Build history of the part. All positions in model axes, mm. A direction names the side the tool comes from. Round coordinates to 2 decimals unless told otherwise and drop trailing zeros. Order: outer loops, then holes, each group sorted by start corner. A loop starts at its lowest first (then second) coordinate and runs counter-clockwise, first axis right, second up. Notation, with made-up numbers: (55, 89) -> (90, 89) arc R23 ccw to (90, 116) -> close; hole circle Ø3 at (29.25, 59.25). An arc over 180 degrees is marked (long way). Use a Markdown table: item, result. Add a question column.
Item 1: Pin check, flat tips, straight feed: pin 1 (3 mm diameter, centred on y = -1.5, z = 4.5, fed in from -X); pin 2 (2 mm diameter, centred on x = 5, z = 4.5, fed in from -Y). Stop position of each tip, or through.
Item 2: Probe L1, parallel to X at y = -1.25, z = 0.75; L2, parallel to X at y = -2.25, z = -1.75; L3, parallel to Z at x = 1, y = -3.5. List the from-to ranges inside material, lowest first.
Item 3: Slice it at A-A, the plane x = -7. Give the cut face in (y, z) (3 decimals).
Item 4: Slice it at C-C, the plane y = -1. State how many separate pieces and enclosed holes the cut face has, plus the area to 3 significant figures.
Item 5: Slice it at B-B, the plane z = 3.75. Give the cut face in (x, y), plus the area to 3 significant figures.
Item 6: 3-axis set-ups, long thin cutter, end or side, ignore diameter. For faces 4 (the face through (-8.24, -1.97, 6.1)), 5 (the face through (-1.35, -3.289, 1.375)), 6 (the face through (-8.223, -1.972, -6.114)): which of +Z, -Z, +X, -X, +Y, -Y reach the whole face in a straight line?
Item 7: Two-plate mould, pull along Z, no slides. Class faces 1 (the face through (-2, -0.5, 1)), 2 (the face through (8.223, -1.972, 6.114)), 3 (the face through (2, -6, 0)): released by +Z, released by -Z, zero draft, split by the parting line, or undercut.
from build123d import *

# Parameters (mm, degrees)
BOSS_EXTRUDE1_DEPTH = 4
BOSS_EXTRUDE1_DRAFT = 1
SHELL1_T            = -0.5
SKETCH2_R           = 2
BOSS_EXTRUDE2_DEPTH = 5.5
BOSS_EXTRUDE2_TAPER = 1.5
CIRPATTERN1_COUNT   = 4
SKETCH4_R           = 1.605977431
CUT_EXTRUDE1_DEPTH  = 5.5
CUT_EXTRUDE1_DRAFT  = 1.5
BOSS_EXTRUDE3_DEPTH = 2.5
BOSS_EXTRUDE4_DEPTH = 2.5


with BuildPart() as part:
    # Sketch1 → Boss-Extrude1 (with draft: the straight prism first)
    with BuildSketch(Plane(origin=(0, 0, 0), x_dir=(1, 0, 0), z_dir=(0, 1, 0))):
        with BuildLine():
            Line((-7.5, -6.375), (7.5, -6.375))
            ThreePointArc((7.5, -6.375), (8.207106781, -6.082106781), (8.5, -5.375))
            Line((8.5, -5.375), (8.5, 5.375))
            ThreePointArc((8.5, 5.375), (8.207106781, 6.082106781), (7.5, 6.375))
            Line((7.5, 6.375), (-7.5, 6.375))
            ThreePointArc((-7.5, 6.375), (-8.207106781, 6.082106781), (-8.5, 5.375))
            Line((-8.5, 5.375), (-8.5, -5.375))
            ThreePointArc((-8.5, -5.375), (-8.207106781, -6.082106781), (-7.5, -6.375))
        make_face()
    extrude(amount=-BOSS_EXTRUDE1_DEPTH)
    # Boss-Extrude1: the draft: its side faces are tilted about the plane it starts from
    boss_extrude1_sides = [part.faces().sort_by_distance(p)[0] for p in [
        (0, -2, 6.375),
        (8.207106781, -2, 6.082106781),
        (8.5, -2, 0),
        (8.207106781, -2, -6.082106781),
        (0, -2, -6.375),
        (-8.207106781, -2, -6.082106781),
        (-8.5, -2, 0),
        (-8.207106781, -2, 6.082106781),
    ]]
    draft(boss_extrude1_sides, Plane(origin=(0, 0, 0), x_dir=(1, 0, 0), z_dir=(0, 1, 0)), BOSS_EXTRUDE1_DRAFT)

    # Shell1
    shell1_openings = [part.faces().sort_by_distance(p)[0] for p in [
        (0, -4, 0),
    ]]
    offset(amount=SHELL1_T, openings=shell1_openings, kind=Kind.INTERSECTION)

    # Sketch2 → Boss-Extrude2 (add)
    with BuildSketch(Plane.XZ.offset(0.5)):
        Circle(SKETCH2_R)
    extrude(amount=BOSS_EXTRUDE2_DEPTH, taper=BOSS_EXTRUDE2_TAPER)

    # Rib1: read off the stored shape, not the designer's step
    # Rib1: loft between two sections, ruled curve by curve
    rib1_from = [
        Edge.make_line((1.982008415, -0.5, 0.267661433), (3, -0.5, 0.25)),
        Edge.make_line((1.982008415, -0.5, -0.267661433), (3, -0.5, -0.25)),
        Edge.make_line((3, -0.5, -0.25), (3, -0.5, 0.25)),
        Edge.make_line((1.982008415, -0.5, -0.267661433), (1.982008415, -0.5, 0.267661433)),
    ]
    rib1_to = [
        Edge.make_line((1.837730654, -6, 0.259611763), (2.391745366, -6, 0.25)),
        Edge.make_line((1.837730654, -6, -0.259611763), (2.391745366, -6, -0.25)),
        Edge.make_line((2.391745366, -6, -0.25), (2.391745366, -6, 0.25)),
        Edge.make_line((1.837730654, -6, -0.259611763), (1.837730654, -6, 0.259611763)),
    ]
    rib1 = Solid(Shell([*[Face.make_surface_from_curves(rib1_from[k], rib1_to[k]) for k in range(4)], Face(Wire(rib1_from)), Face(Wire(rib1_to))]))
    add(rib1)

    # CirPattern1: Rib1 ×4 about axis
    cirpattern1_axis = Axis((0, 0, 0), (0, 1, 0))
    for i in range(1, CIRPATTERN1_COUNT):
        add(rib1.rotate(cirpattern1_axis, i * 360 / CIRPATTERN1_COUNT))


with BuildPart() as cut_extrude1_tool:
    # Sketch4 → Cut-Extrude1 (with draft: the straight prism first)
    with BuildSketch(Plane.XZ.offset(6)):
        Circle(SKETCH4_R)
    extrude(amount=-CUT_EXTRUDE1_DEPTH)
    # Cut-Extrude1: the draft: its side faces are tilted about the plane it starts from
    cut_extrude1_sides = [cut_extrude1_tool.faces().sort_by_distance(p)[0] for p in [
        (-1.605977431, -3.25, 0),
    ]]
    draft(cut_extrude1_sides, Plane.XZ.offset(6), CUT_EXTRUDE1_DRAFT)


with BuildPart() as part_1:
    add(part.part)

    # Cut-Extrude1: cut by cut_extrude1_tool
    add(cut_extrude1_tool.part, mode=Mode.SUBTRACT)

    # Sketch5 → Boss-Extrude3 (add, symmetric)
    with BuildSketch(Plane(origin=(0, 0, 0), x_dir=(0, 0, -1), z_dir=(1, 0, 0))):
        Polygon((6.44482026, -4), (6.40991013, -2), (6.70991013, -2), align=None)
        Polygon((-6.70991013, -2), (-6.44482026, -4), (-6.40991013, -2), align=None)
    extrude(amount=BOSS_EXTRUDE3_DEPTH, both=True)

    # Sketch6 → Boss-Extrude4 (add, symmetric)
    with BuildSketch(Plane.XY):
        Polygon((8.56982026, -4), (8.53491013, -2), (8.83491013, -2), align=None)
        Polygon((-8.83491013, -2), (-8.56982026, -4), (-8.53491013, -2), align=None)
    extrude(amount=BOSS_EXTRUDE4_DEPTH, both=True)


solid = part_1.part
Check sheet entries:
| question | item | result |
|---|---|---|
| 1 | pin 1 | x = -8.55 |
| 1 | pin 2 | y = -0.5 |
| 2 | L1 | -8.52 to -8.02, -1.83 to -1.56, 1.56 to 1.83, 8.02 to 8.52 |
| 2 | L2 | -8.8 to -8.04, -0.87 to 0.87, 8.04 to 8.8 |
| 2 | L3 | -6.51 to -5.94, -1.64 to -1.34, 1.34 to 1.64, 5.94 to 6.51 |
| 3 | outline | (-4, -6.445) -> (0, -6.375) -> (0, 6.375) -> (-4, 6.445) -> (-4, 5.945) -> (-0.5, 5.884) -> (-0.5, -5.884) -> (-4, -5.945) -> close |
| 4 | separate pieces | 2 |
| 4 | enclosed holes | 2 |
| 4 | area | 33.1 mm2 |
| 5 | outline | (-8.57, -4) -> (-8.07, -4) -> (-8.01, -0.5) -> (8.01, -0.5) -> (8.07, -4) -> (8.57, -4) -> (8.5, 0) -> (-8.5, 0) -> close |
| 5 | area | 12.0 mm2 |
| 6 | face 4 | +Z, -X, +Y |
| 6 | face 5 | -Y |
| 6 | face 6 | -Z, -X, +Y |
| 7 | face 1 | undercut |
| 7 | face 2 | released by +Z |
| 7 | face 3 | zero draft |
